```python
from build123d import *

# Parameters (mm, degrees)
SKETCH1_W            = 42
SKETCH1_H            = 42
SKETCH1_R            = 11
BOSS_EXTRUDE1_DEPTH  = 1.5875
M3_CLEARANCE_HOLE1_D = 3.2
SKETCH4_W            = 5
SKETCH4_H            = 42
SKETCH4_W_2          = 10
SKETCH4_H_2          = 28
BOSS_EXTRUDE2_DEPTH  = 3.175
SKETCH5_W            = 7
SKETCH5_H            = 0.7
BOSS_EXTRUDE3_DEPTH  = 3.175
FILLET1_R            = 1


with BuildPart() as part:
    # Sketch1 → Boss-Extrude1 (new, symmetric)
    with BuildSketch(Plane(origin=(0, 0, 0), x_dir=(1, 0, 0), z_dir=(0, 1, 0))):
        Rectangle(SKETCH1_W, SKETCH1_H)
        with Locations(Location((0, 0, 0), (0, 0, 270))):
            Circle(SKETCH1_R, mode=Mode.SUBTRACT)
    extrude(amount=BOSS_EXTRUDE1_DEPTH, both=True)

    # M3 Clearance Hole1 (through all)
    with Locations(Plane(origin=(0, 1.5875, 0), x_dir=(1, 0, 0), z_dir=(0, 1, 0))):
        with Locations((-15.5, 15.5), (15.5, 15.5), (15.5, -15.5), (-15.5, -15.5)):
            Hole(M3_CLEARANCE_HOLE1_D / 2)

    # Sketch4 → Boss-Extrude2 (add)
    # profile 1 of 4: a face of its own
    with BuildSketch(Plane(origin=(0, 1.5875, 0), x_dir=(1, 0, 0), z_dir=(0, 1, 0))):
        with BuildLine():
            Line((1.6, -24), (1.6, -28.7))
            Line((1.6, -28.7), (14, -28.7))
            Line((14, -28.7), (14, -21))
            Line((14, -21), (-19, -21))
            Line((-19, -21), (-19, -28.7))
            Line((-19, -28.7), (-1.6, -28.7))
            Line((-1.6, -28.7), (-1.6, -24))
            ThreePointArc((-1.6, -24), (0, -22.4), (1.6, -24))
        make_face()
    # profile 2 of 4: a face of its own
    with BuildSketch(Plane(origin=(0, 1.5875, 0), x_dir=(1, 0, 0), z_dir=(0, 1, 0))):
        with Locations((-23.5, 0)):
            Rectangle(SKETCH4_W, SKETCH4_H)
    # profile 3 of 4: a face of its own
    with BuildSketch(Plane(origin=(0, 1.5875, 0), x_dir=(1, 0, 0), z_dir=(0, 1, 0))):
        with BuildLine():
            Line((1.6, 28.7), (14, 28.7))
            Line((14, 28.7), (14, 21))
            Line((14, 21), (-19, 21))
            Line((-19, 21), (-19, 28.7))
            Line((-19, 28.7), (-1.6, 28.7))
            Line((-1.6, 28.7), (-1.6, 24))
            ThreePointArc((-1.6, 24), (0, 22.4), (1.6, 24))
            Line((1.6, 24), (1.6, 28.7))
        make_face()
    # profile 4 of 4: a face of its own
    with BuildSketch(Plane(origin=(0, 1.5875, 0), x_dir=(1, 0, 0), z_dir=(0, 1, 0))):
        with Locations((26, 0)):
            Rectangle(SKETCH4_W_2, SKETCH4_H_2)
        with BuildLine():
            Line((27.6, 1.5), (27.6, -1.5))
            ThreePointArc((27.6, -1.5), (26, -3.1), (24.4, -1.5))
            Line((24.4, -1.5), (24.4, 1.5))
            ThreePointArc((24.4, 1.5), (26, 3.1), (27.6, 1.5))
        make_face(mode=Mode.SUBTRACT)
    extrude(amount=-BOSS_EXTRUDE2_DEPTH)

    # Sketch5 → Boss-Extrude3 (add)
    with BuildSketch(Plane(origin=(0, 1.5875, 0), x_dir=(1, 0, 0), z_dir=(0, 1, 0))):
        Polygon((21, 14), (31, 14), (31, 21.7), (24, 21.7), (24, 28.7), (14, 28.7), (14, 21), (21, 21), align=None)
        Polygon((31, -14), (21, -14), (21, -21), (14, -21), (14, -28.7), (24, -28.7), (24, -21.7), (31, -21.7), align=None)
        with Locations((-22.5, -21.35)):
            Rectangle(SKETCH5_W, SKETCH5_H)
        with Locations((-22.5, 21.35)):
            Rectangle(SKETCH5_W, SKETCH5_H)
    extrude(amount=-BOSS_EXTRUDE3_DEPTH)

    # Fillet1
    fillet1_edges = [part.edges().sort_by_distance(p)[0] for p in [
        (-26, 0, 21.7),
        (31, 0, -21.7),
        (-19, 0, -21.7),
        (24, 0, -28.7),
        (24, 0, -21.7),
        (31, 0, 21.7),
        (24, 0, 21.7),
        (24, 0, 28.7),
        (-19, 0, 21.7),
        (-26, 0, -21.7),
        (-1.6, 0, 28.7),
        (-19, 0, 28.7),
        (1.6, 0, 28.7),
        (1.6, 0, -28.7),
        (-19, 0, -28.7),
        (-1.6, 0, -28.7),
    ]]
    fillet(fillet1_edges, radius=FILLET1_R)


solid = part.part
```
Check sheet for the modelled part. Datum: model origin and axes. Units: mm. A direction names the side the tool comes from. Coordinates: 2 decimals unless noted, no trailing zeros. Order: outer loops, then holes, each group sorted by start corner. A loop starts at its lowest first (then second) coordinate and runs counter-clockwise, first axis right, second up. Notation, with made-up numbers: (10, 68.5) -> (65, 68.5) arc R12 ccw to (65, 89.5) -> close; hole circle Ø1 at (68.25, 43). An arc over 180 degrees is marked (long way). Write each question's results on one line, items separated by ' | '. Start each with the question number.
1) Section check C-C (x = 26). Enter the section's corners in (y, z).
2) Section check B-B (z = 15.5). Enter the section's corners in (x, y).
3) Section check A-A (x = -15.5). Enter the section's corners in (y, z).
4) Section check D-D (z = -8). Enter the section's corners in (x, y).
5) Set-up check for faces 4 (the face through (-23, 0, 21.7)), 5 (the face through (26, 0, 3.1)), 6 (the face through (24, 0, 25)): record each of +Z, -Z, +X, -X, +Y, -Y from which the full face is reachable in a straight line by a thin tool's end or side.
6) Depth check by flat-ended pin: pin 1 (1 mm diameter, centred on y = 0.5, z = -25.5, fed in from -X); pin 2 (5 mm diameter, centred on x = -7.5, z = -2.5, fed in from +Y); pin 3 (1 mm diameter, centred on y = -0.5, z = -25.5, fed in from +X); pin 4 (1.6 mm diameter, centred on x = -23.5, y = 0, fed in from -Z). Enter the tip coordinate at first touch or a pass-through.
7) Draft check along X on faces 1 (the face through (2, 1.588, -13)), 2 (the face through (-10.74, -0.02, -2.38)), 3 (the face through (-19, 0, -25)). Enter one of: pulls with the +X half, pulls with the -X half, needs draft (parallel to the pull), parting line crosses it, or undercut.
8) Material ranges on line 1 along X through (y, z) = (0.1, -15.5); line 2 along Z through (x, y) = (15.5, 0.85); line 3 along X through (y, z) = (-0.35, 4), recorded low to high.
Checked values:
1) outline: (-1.59, -21.7) -> (1.59, -21.7) -> (1.59, -3.1) -> (-1.59, -3.1) -> close; (-1.59, 3.1) -> (1.59, 3.1) -> (1.59, 21.7) -> (-1.59, 21.7) -> close
2) outline: (-26, -1.59) -> (-17.1, -1.59) -> (-17.1, 1.59) -> (-26, 1.59) -> close; (-13.9, -1.59) -> (13.9, -1.59) -> (13.9, 1.59) -> (-13.9, 1.59) -> close; (17.1, -1.59) -> (31, -1.59) -> (31, 1.59) -> (17.1, 1.59) -> close
3) outline: (-1.59, -28.7) -> (1.59, -28.7) -> (1.59, -17.1) -> (-1.59, -17.1) -> close; (-1.59, -13.9) -> (1.59, -13.9) -> (1.59, 13.9) -> (-1.59, 13.9) -> close; (-1.59, 17.1) -> (1.59, 17.1) -> (1.59, 28.7) -> (-1.59, 28.7) -> close
4) outline: (-26, -1.59) -> (-7.55, -1.59) -> (-7.55, 1.59) -> (-26, 1.59) -> close; (7.55, -1.59) -> (31, -1.59) -> (31, 1.59) -> (7.55, 1.59) -> close
5) face 4: +Z, -X, +Y, -Y | face 5: +Y, -Y | face 6: +Z, +X, +Y, -Y
6) pin 1: x = -19 | pin 2: through | pin 3: x = 24 | pin 4: z = -21.7
7) face 1: needs draft | face 2: undercut | face 3: pulls with the -X half
8) line 1: -26 to -17.1, -13.9 to 13.9, 17.1 to 31 | line 2: -28.7 to -17.1, -13.9 to 13.9, 17.1 to 28.7 | line 3: -26 to -10.25, 10.25 to 31
